Source: three-view drawing plus pictorial views. Frame: mm from the lowest corner of the part. A direction names the side the tool comes from. Give positions to 0.01 mm unless a question says otherwise; leave off trailing zeros. Loops run counter-clockwise (first coordinate to the right, second up) from the corner with the lowest first, then second, coordinate; pieces in that order, holes last. Notation, with made-up numbers: (65, 70.5) -> (86, 70.5) arc R31 cw to (86, 100.5) -> close; hole circle Ø9 at (74.5, 0). An arc over 180 degrees is marked (long way). Put each result on its own line as item: value.
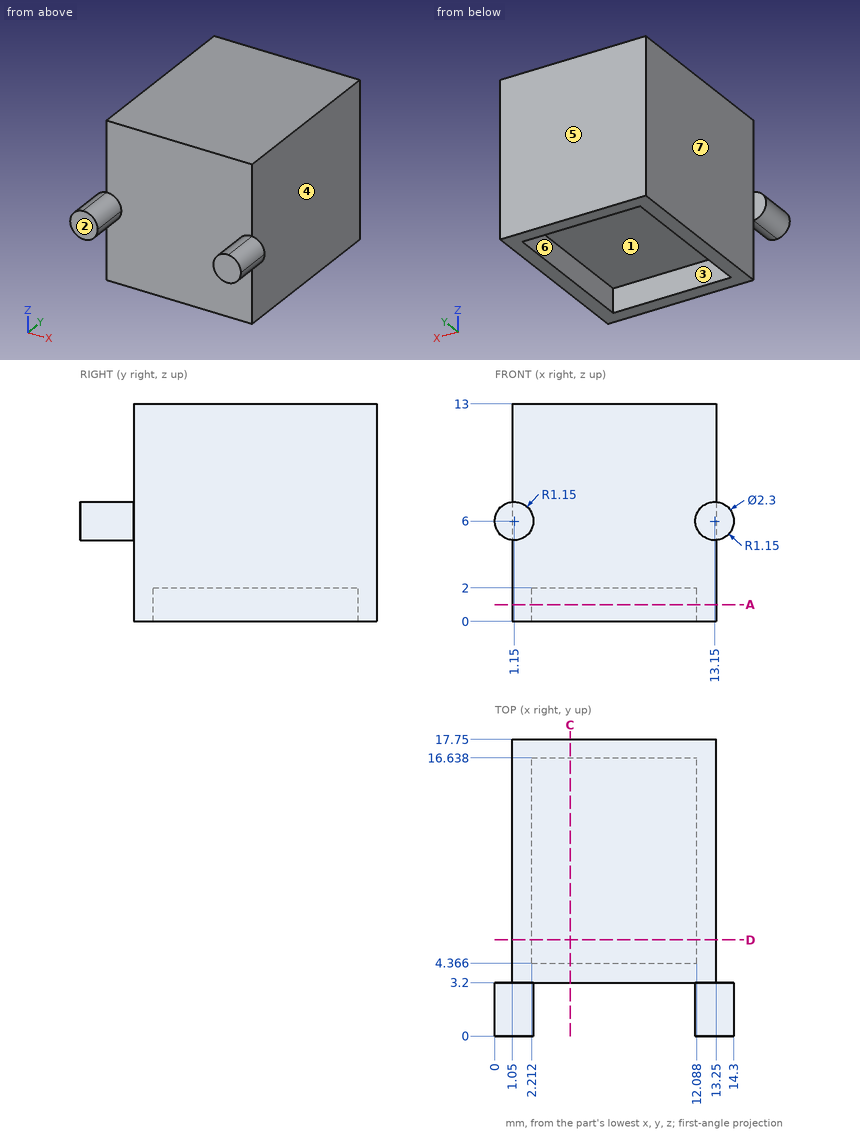
(1) First-contact query: P1, Ø0.6, axis at x = 6.5, z = 0.5, coming from the -Y side; P2, Ø0.8, axis at x = 0.5, z = 6.5, coming from the +Y side; P3, Ø1, axis at y = 10, z = 1, coming from the +X side. Flat tips, straight axial feed; report the tip coordinate or a pass-through.
Calculated:
P1: stops at y = 3.2
P2: stops at y = 3.2
P3: stops at x = 13.25
(2) Draft query along Y for the marked faces 1, 2, 3 and 4. Return one class per face: released by +Y, released by -Y, zero draft, split by the parting line, or undercut.
Calculated:
face 1: undercut
face 2: released by -Y
face 3: undercut
face 4: zero draft
(3) Section D-D on y = 5.75. Return loops of the section in (x, z).
Calculated:
outline: (1.05, 0) -> (2.21, 0) -> (2.21, 2) -> (12.09, 2) -> (12.09, 0) -> (13.25, 0) -> (13.25, 13) -> (1.05, 13) -> close
(4) Section A-A on z = 1. Return loops of the section in (x, y).
Calculated:
outline: (1.05, 3.2) -> (13.25, 3.2) -> (13.25, 17.75) -> (1.05, 17.75) -> close; hole (2.21, 4.37) -> (12.09, 4.37) -> (12.09, 16.64) -> (2.21, 16.64) -> close
(5) Line query: probe 1 along Z at (x, y) = (11.5, 7); probe 2 along Y at (x, z) = (10.5, 2.5); probe 3 along X at (y, z) = (3.75, 3.25). Output: solid intervals per line, ascending. Write a range as from..to.
Calculated:
probe 1: z = 2..13
probe 2: y = 3.2..17.75
probe 3: x = 1.05..13.25
(6) Reachability of the marked faces 5, 6 and 7 from +Z, -Z, +X, -X, +Y, -Y: full face, straight path, thin tool, end or side. Return the list, or none.
Calculated:
face 5: +Z, -Z, +X, -X, +Y
face 6: -Z
face 7: +Z, -Z, -X, +Y
(7) Section C-C on x = 4.5. Return loops of the section in (y, z), then the cut area to 3 significant figures.
Calculated:
outline: (3.2, 0) -> (4.37, 0) -> (4.37, 2) -> (16.64, 2) -> (16.64, 0) -> (17.75, 0) -> (17.75, 13) -> (3.2, 13) -> close
area: 165 mm²
